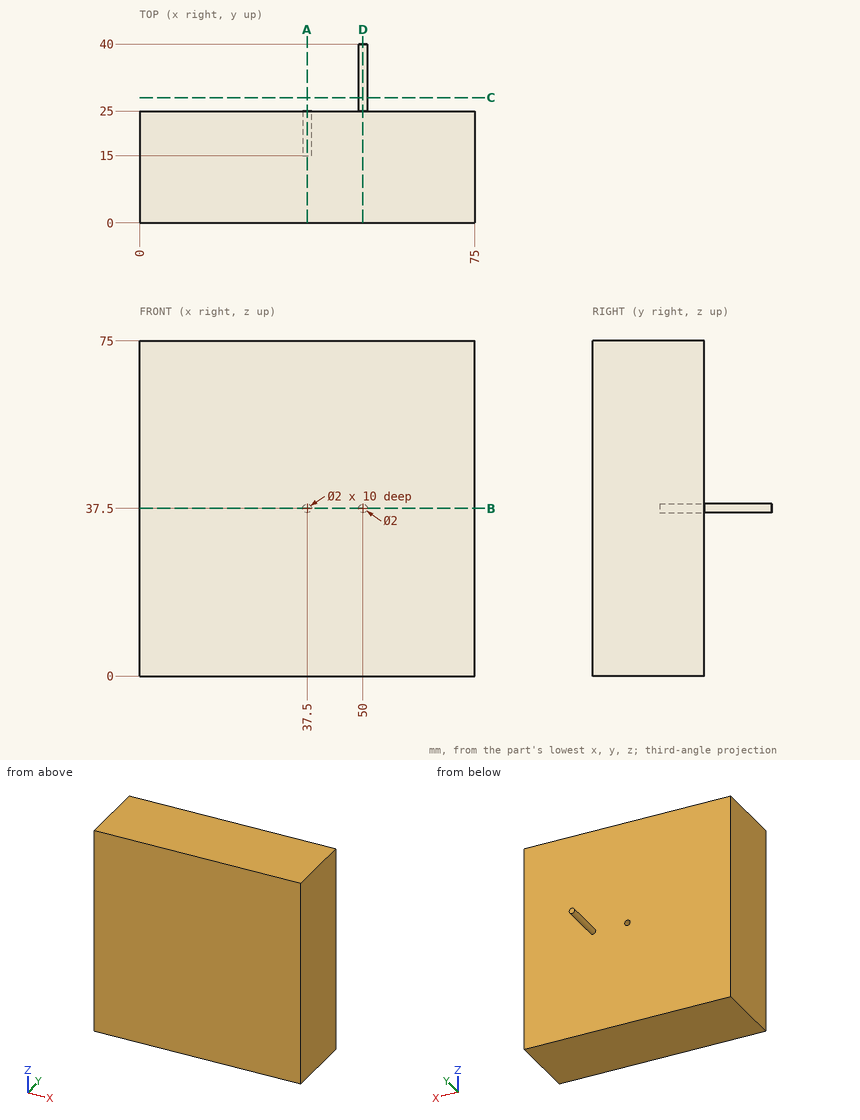
The drawing under review shows one solid part. Ordinate dimensions are in mm from its lowest x, y, z. Give positions to 0.01 mm unless a question says otherwise; leave off trailing zeros. Write each loop counter-clockwise with the first axis right and the second up, starting at its lowest first coordinate (ties: lowest second). Pieces come first, ordered by that corner, then holes.
1. For P1, Ø1.6, axis at x = 37.5, z = 37.5, coming from the +Y side, flat-tipped, find the tip position at first contact; note if it passes through.
2. Add section A-A, the plane x = 37.5. Write out the cut boundary in (y, z), plus the area to 4 significant figures.
3. Add section C-C, the plane y = 28. Write out the cut boundary in (x, z), plus the area to 3 significant figures.
4. Add section B-B, the plane z = 37.5. Write out the cut boundary in (x, y), plus the area to 4 significant figures.
5. Wall thickness on L1, parallel to Z at x = 37.5, y = 21.5; L2, parallel to Y at x = 23, z = 22; L3, parallel to X at y = 21, z = 37: over which ranges is each line inside the solid? List them lowest first.
6. Add section D-D, the plane x = 50. Write out the cut boundary in (y, z), plus the area to 4 significant figures.
Worked answers:
1. P1: stops at y = 15
2. outline: (0, 0) - (25, 0) - (25, 36.5) - (15, 36.5) - (15, 38.5) - (25, 38.5) - (25, 75) - (0, 75) - close
2. area: 1,855 mm2
3. outline: circle Ø2 at (50, 37.5)
3. area: 3.14 mm2
4. outline: (0, 0) - (75, 0) - (75, 25) - (51, 25) - (51, 40) - (49, 40) - (49, 25) - (38.5, 25) - (38.5, 15) - (36.5, 15) - (36.5, 25) - (0, 25) - close
4. area: 1,885 mm2
5. L1: z = 0 to 36.5, 38.5 to 75
5. L2: y = 0 to 25
5. L3: x = 0 to 36.63, 38.37 to 75
6. outline: (0, 0) - (25, 0) - (25, 36.5) - (40, 36.5) - (40, 38.5) - (25, 38.5) - (25, 75) - (0, 75) - close
6. area: 1,905 mm2
